from build123d import *

# Parameters (mm, degrees)
SKETCH7_W          = 1.5875
SKETCH7_H          = 7.62
CUT_EXTRUDE1_DEPTH = 0.0254


with BuildPart() as part:
    # Sketch1 → Complete_Ball (revolve)
    with BuildSketch(Plane.XY):
        with BuildLine():
            Line((0, 12.7), (0, -12.7))
            ThreePointArc((0, -12.7), (12.7, 0), (0, 12.7))
        make_face()
    revolve(axis=Axis((0, 13.965019531, 0), (0, -1, 0)))

    # Sketch7 → Ball_w_concentric_hole (revolve, cut)
    with BuildSketch(Plane.XY):
        with Locations((0.79375, -8.89)):
            Rectangle(SKETCH7_W, SKETCH7_H)
    revolve(axis=Axis((0, -6.726898043, 0), (0, 1, 0)), mode=Mode.SUBTRACT)

    # Sketch9 → Cut-Extrude1 (cut)
    with BuildSketch(Plane.XZ.offset(5.08)):
        with BuildLine():
            add(Edge.make_bspline(
                [(0.308076994, -0.030373732), (0.324538713, -0.034024291), (0.356530602, -0.041118827), (0.402477662, -0.054290859), (0.445054282, -0.069285046), (0.484732885, -0.085294373), (0.521280558, -0.103036208), (0.554555606, -0.122564651), (0.584482781, -0.143830699), (0.602480105, -0.159466562), (0.611281283, -0.167112921)],
                knots=[0, 0, 0, 0, 1.202298385, 2.336560135, 3.406084711, 4.420247637, 5.386399354, 6.300522109, 7.168909389, 8, 8, 8, 8], degree=3))
            add(Edge.make_bspline(
                [(0.611281283, -0.167112921), (0.622417749, -0.178075677), (0.644400951, -0.199715976), (0.67281694, -0.235522748), (0.696753104, -0.273154409), (0.716536823, -0.312521351), (0.731766785, -0.353857034), (0.742939599, -0.39692676), (0.749363419, -0.441811935), (0.750162969, -0.472278831), (0.750568408, -0.487728101)],
                knots=[0, 0, 0, 0, 1.040892545, 2.054704896, 3.038886078, 4.009403739, 4.985637774, 5.96968326, 6.970459233, 8, 8, 8, 8], degree=3))
            add(Edge.make_bspline(
                [(0.750568408, -0.487728101), (0.749580677, -0.511480749), (0.747596123, -0.559204719), (0.728910303, -0.629570582), (0.700367842, -0.698612498), (0.660350876, -0.764646818), (0.611443791, -0.826373993), (0.551760396, -0.878883273), (0.484387528, -0.923101532), (0.421448289, -0.952346751), (0.365407997, -0.970620061), (0.317719104, -0.98275638), (0.264926091, -0.993624769), (0.20667372, -1.001054176), (0.143434911, -1.008194794), (0.07484539, -1.01250787), (0.001081213, -1.015688606), (-0.049903845, -1.015893946), (-0.076236566, -1.016)],
                knots=[0, 0, 0, 0, 1.028770293, 2.067011775, 3.138033473, 4.261901228, 5.406207792, 6.541562624, 7.694800496, 8.892876887, 9.539626609, 10.250184141, 11.027081459, 11.876550478, 12.796927842, 13.788050093, 14.85757392, 16, 16, 16, 16], degree=3))
            Line((-0.076236566, -1.016), (-0.988822024, -1.016))
            Line((-0.988822024, -1.016), (-0.988822024, -0.961644049))
            Line((-0.988822024, -0.961644049), (-0.917904495, -0.961644049))
            add(Edge.make_bspline(
                [(-0.917904495, -0.961644049), (-0.908402664, -0.961432941), (-0.890024832, -0.961024629), (-0.863622385, -0.956950597), (-0.839065748, -0.951375967), (-0.816950335, -0.942204208), (-0.796626646, -0.931084721), (-0.778261022, -0.917590019), (-0.762272466, -0.901062238), (-0.753405479, -0.88858522), (-0.74889146, -0.882233402)],
                knots=[0, 0, 0, 0, 1.166786496, 2.256723755, 3.277842578, 4.25348796, 5.187934752, 6.120436128, 7.043148905, 8, 8, 8, 8], degree=3))
            add(Edge.make_bspline(
                [(-0.74889146, -0.882233402), (-0.746190352, -0.877347431), (-0.740363736, -0.866807802), (-0.734346678, -0.84805755), (-0.728780995, -0.826107168), (-0.724762233, -0.800356427), (-0.721378545, -0.77103352), (-0.718963551, -0.738021693), (-0.71713277, -0.701491854), (-0.717073307, -0.675994887), (-0.717042269, -0.662686318)],
                knots=[0, 0, 0, 0, 0.597321695, 1.288494999, 2.101981578, 3.025155317, 4.079375286, 5.266669335, 6.573292293, 8, 8, 8, 8], degree=3))
            Line((-0.717042269, -0.662686318), (-0.717042269, 0.587500555))
            add(Edge.make_bspline(
                [(-0.717042269, 0.587500555), (-0.717020857, 0.602227129), (-0.716980065, 0.63028246), (-0.719451119, 0.670192763), (-0.721936908, 0.705972397), (-0.726817478, 0.737387607), (-0.732121451, 0.764688921), (-0.738568219, 0.7877891), (-0.747095316, 0.806473529), (-0.754139821, 0.816751719), (-0.757384577, 0.821485937)],
                knots=[0, 0, 0, 0, 1.467983741, 2.79662948, 3.986363477, 5.042318655, 5.964098798, 6.759038926, 7.428403245, 8, 8, 8, 8], degree=3))
            add(Edge.make_bspline(
                [(-0.757384577, 0.821485937), (-0.766968382, 0.831548203), (-0.786306937, 0.851852213), (-0.824785442, 0.872201997), (-0.869332734, 0.884203522), (-0.901116145, 0.885678948), (-0.917904495, 0.886458285)],
                knots=[0, 0, 0, 0, 0.927123666, 1.870784184, 2.875324672, 4, 4, 4, 4], degree=3))
            Line((-0.917904495, 0.886458285), (-0.988822024, 0.886458285))
            Line((-0.988822024, 0.886458285), (-0.988822024, 0.940814236))
            Line((-0.988822024, 0.940814236), (-0.162866363, 0.940814236))
            add(Edge.make_bspline(
                [(-0.162866363, 0.940814236), (-0.126188539, 0.940513422), (-0.056725795, 0.939943722), (0.041752121, 0.932910915), (0.129010541, 0.922793404), (0.182730464, 0.91105738), (0.207858209, 0.905567799)],
                knots=[0, 0, 0, 0, 1.179035714, 2.232931189, 3.173445281, 4, 4, 4, 4], degree=3))
            add(Edge.make_bspline(
                [(0.207858209, 0.905567799), (0.225058291, 0.900995857), (0.258662627, 0.892063511), (0.306862604, 0.874872481), (0.35200904, 0.855362596), (0.394161004, 0.833417302), (0.432870067, 0.808543943), (0.468965178, 0.781808256), (0.501653259, 0.752055301), (0.530912052, 0.719772753), (0.556715696, 0.685606681), (0.580062927, 0.650467371), (0.598866319, 0.613375247), (0.614986078, 0.57548153), (0.626598012, 0.536066061), (0.635806285, 0.495707281), (0.640869134, 0.453863359), (0.641524814, 0.425577459), (0.641856506, 0.41126837)],
                knots=[0, 0, 0, 0, 1.197163213, 2.33893505, 3.43955965, 4.504702612, 5.532566955, 6.532694419, 7.523891994, 8.501634608, 9.459882266, 10.403051993, 11.336018195, 12.25408421, 13.170072591, 14.09679423, 15.037218469, 16, 16, 16, 16], degree=3))
            add(Edge.make_bspline(
                [(0.641856506, 0.41126837), (0.640988305, 0.386966428), (0.639277347, 0.339074706), (0.622358228, 0.269582217), (0.595666689, 0.204017494), (0.565112824, 0.152992911), (0.535110113, 0.115449663), (0.510556404, 0.08830852), (0.482805357, 0.063927102), (0.452810586, 0.041062695), (0.420086682, 0.020541755), (0.38522035, 0.001209477), (0.347651311, -0.015759261), (0.321445222, -0.025436955), (0.308076994, -0.030373732)],
                knots=[0, 0, 0, 0, 1.471082931, 2.899056279, 4.307818116, 5.751614296, 6.484736272, 7.219614112, 7.967209451, 8.720692231, 9.503935749, 10.306636219, 11.136182697, 12, 12, 12, 12], degree=3))
        make_face()
        with BuildLine():
            add(Edge.make_bspline(
                [(-0.445262514, 0.037995862), (-0.426327321, 0.034656251), (-0.386080053, 0.027557818), (-0.321529386, 0.021144961), (-0.249825238, 0.017428628), (-0.199675095, 0.016991416), (-0.173482759, 0.016763069)],
                knots=[0, 0, 0, 0, 0.844887106, 1.795830451, 2.848809897, 4, 4, 4, 4], degree=3))
            add(Edge.make_bspline(
                [(-0.173482759, 0.016763069), (-0.156495387, 0.016960654), (-0.123639547, 0.017342808), (-0.076026849, 0.019288173), (-0.031719973, 0.023285242), (0.00930446, 0.028009349), (0.047066576, 0.035115731), (0.08167708, 0.042721005), (0.112945821, 0.052723303), (0.149614447, 0.066940798), (0.19007552, 0.088916151), (0.23035913, 0.122823227), (0.261457989, 0.163456789), (0.282889969, 0.210155805), (0.296731598, 0.260777518), (0.308199203, 0.31345399), (0.314500353, 0.368508228), (0.315309667, 0.405874992), (0.3157208, 0.424857357)],
                knots=[0, 0, 0, 0, 1.091830023, 2.111744693, 3.061402081, 3.95056914, 4.764258185, 5.530001833, 6.226288629, 6.871621508, 8.056545267, 9.166642, 10.231067328, 11.317616446, 12.446050905, 13.598649409, 14.780110772, 16, 16, 16, 16], degree=3))
            add(Edge.make_bspline(
                [(0.3157208, 0.424857357), (0.315274183, 0.439594324), (0.314394441, 0.468623136), (0.308579089, 0.511424009), (0.297616446, 0.552413229), (0.283341565, 0.591889551), (0.264856225, 0.629856323), (0.24190265, 0.6657694), (0.214734501, 0.700054926), (0.1840394, 0.732629931), (0.149194905, 0.76249929), (0.110236379, 0.788477557), (0.067684677, 0.810609885), (0.021216663, 0.82849277), (-0.028831328, 0.842453754), (-0.082873755, 0.85205292), (-0.140507573, 0.858047973), (-0.180261974, 0.858862407), (-0.200660735, 0.85928031)],
                knots=[0, 0, 0, 0, 0.932104058, 1.836054539, 2.724128921, 3.610577454, 4.48739039, 5.388899496, 6.300486582, 7.250348221, 8.215526472, 9.196272454, 10.205292906, 11.242666987, 12.339557976, 13.48617357, 14.710106481, 16, 16, 16, 16], degree=3))
            add(Edge.make_bspline(
                [(-0.200660735, 0.85928031), (-0.222755045, 0.858845399), (-0.265893392, 0.857996252), (-0.32895856, 0.852174222), (-0.388604371, 0.84167089), (-0.426645356, 0.831254772), (-0.445262514, 0.826157152)],
                knots=[0, 0, 0, 0, 1.070391011, 2.089899941, 3.065202048, 4, 4, 4, 4], degree=3))
            Line((-0.445262514, 0.826157152), (-0.445262514, 0.037995862))
        make_face(mode=Mode.SUBTRACT)
        with BuildLine():
            add(Edge.make_bspline(
                [(-0.445262514, -0.894973078), (-0.417443506, -0.901131169), (-0.362095565, -0.913383138), (-0.278646345, -0.925338098), (-0.195705669, -0.932903229), (-0.140658937, -0.933945707), (-0.113181626, -0.934466073)],
                knots=[0, 0, 0, 0, 1.019899824, 2.029164851, 3.016231376, 4, 4, 4, 4], degree=3))
            add(Edge.make_bspline(
                [(-0.113181626, -0.934466073), (-0.091929976, -0.934252226), (-0.050751607, -0.933837863), (0.009069282, -0.927437289), (0.065096664, -0.918561989), (0.117145516, -0.905172654), (0.165579696, -0.88891324), (0.209737927, -0.867987195), (0.25019028, -0.843565692), (0.286693969, -0.815673306), (0.318630006, -0.784579101), (0.347205512, -0.752213582), (0.370951573, -0.71762533), (0.390803655, -0.681461485), (0.405596026, -0.643095371), (0.41676876, -0.603336191), (0.423256869, -0.561547228), (0.424035612, -0.533188423), (0.424432702, -0.518727979)],
                knots=[0, 0, 0, 0, 1.335369974, 2.58748639, 3.778398001, 4.898614871, 5.962444548, 6.985554789, 7.963871145, 8.928614683, 9.866425566, 10.762210136, 11.638554271, 12.498661649, 13.349744001, 14.217688406, 15.091181162, 16, 16, 16, 16], degree=3))
            add(Edge.make_bspline(
                [(0.424432702, -0.518727979), (0.4235265, -0.499567493), (0.421710444, -0.461169303), (0.409685349, -0.404035632), (0.388218739, -0.348651871), (0.359964971, -0.294377764), (0.322780244, -0.243092717), (0.275077564, -0.197879287), (0.218738662, -0.157870999), (0.15288954, -0.124748012), (0.078754411, -0.097458162), (-0.003925713, -0.078132811), (-0.094744496, -0.066773569), (-0.158019387, -0.065455602), (-0.19089365, -0.064770857)],
                knots=[0, 0, 0, 0, 0.80426076, 1.611762754, 2.437163379, 3.29025987, 4.174362993, 5.081949637, 6.03643416, 7.064744133, 8.166225842, 9.344998398, 10.620602567, 12, 12, 12, 12], degree=3))
            add(Edge.make_bspline(
                [(-0.19089365, -0.064770857), (-0.205191428, -0.064684482), (-0.232799059, -0.0645177), (-0.272567725, -0.065669626), (-0.309100885, -0.066295208), (-0.351293058, -0.06804369), (-0.396516564, -0.070242075), (-0.430284502, -0.075571351), (-0.445262514, -0.077935189)],
                knots=[0, 0, 0, 0, 1.009225997, 1.948718216, 2.808291512, 3.588270035, 4.930259813, 6, 6, 6, 6], degree=3))
            Line((-0.445262514, -0.077935189), (-0.445262514, -0.894973078))
        make_face(mode=Mode.SUBTRACT)
    extrude(amount=-CUT_EXTRUDE1_DEPTH, mode=Mode.SUBTRACT)


solid = part.part
Can you work these out from the model? Positions are in its coordinate system, mm. Give positions to 0.01 mm unless a question says otherwise; leave off trailing zeros. Loops run counter-clockwise (first coordinate to the right, second up) from the corner with the lowest first, then second, coordinate; pieces in that order, holes last. Notation, with made-up numbers: (18, 77.25) - (34, 77.25) arc R36 cw to (34, 116.25) - close; hole circle Ø7 at (35.25, 23.25). An arc over 180 degrees is marked (long way). Answer as a JSON object with one key per item and string values.
Q1. Imagine slicing it at A-A on y = -10.5. Write out the boundary of the cut face in (x, z) (1 decimal), plus the area to 3 significant figures.
Geometry says:
{"outline": "circle Ø14.3 at (0, 0); hole circle Ø3.2 at (0, 0)", "area": "152 mm²"}
Q2. If I drill on L1, parallel to Z at x = 0, y = -7.25; L2, parallel to X at y = -10.75, z = 0; L3, parallel to X at y = -10.25, z = 0, over which ranges is the centre line in solid material (lowest first)?
Geometry says:
{"L1": "-10.43 to -1.59, 1.59 to 10.43", "L2": "-6.76 to -1.59, 1.59 to 6.76", "L3": "-7.5 to -1.59, 1.59 to 7.5"}
Q3. Imagine slicing it at B-B on x = -2.25. Write out the boundary of the cut face in (y, z).
Geometry says:
{"outline": "circle Ø25 at (0, 0)"}
Q4. Imagine slicing it at C-C on z = -7. Write out the boundary of the cut face in (x, y), plus the area to 3 significant figures.
Geometry says:
{"outline": "circle Ø21.19 at (0, 0)", "area": "353 mm²"}
Q5. Will these pins go through, and if not, where does the flat tip stop? P1, Ø3, axis at y = 3, z = 7.5, coming from the -X side; P2, Ø6, axis at y = 0, z = -9, coming from the +X side; P3, Ø12, axis at y = -0.5, z = 8, coming from the +X side.
Geometry says:
{"P1": "x = -10.86", "P2": "x = 11.19", "P3": "x = 12.54"}
